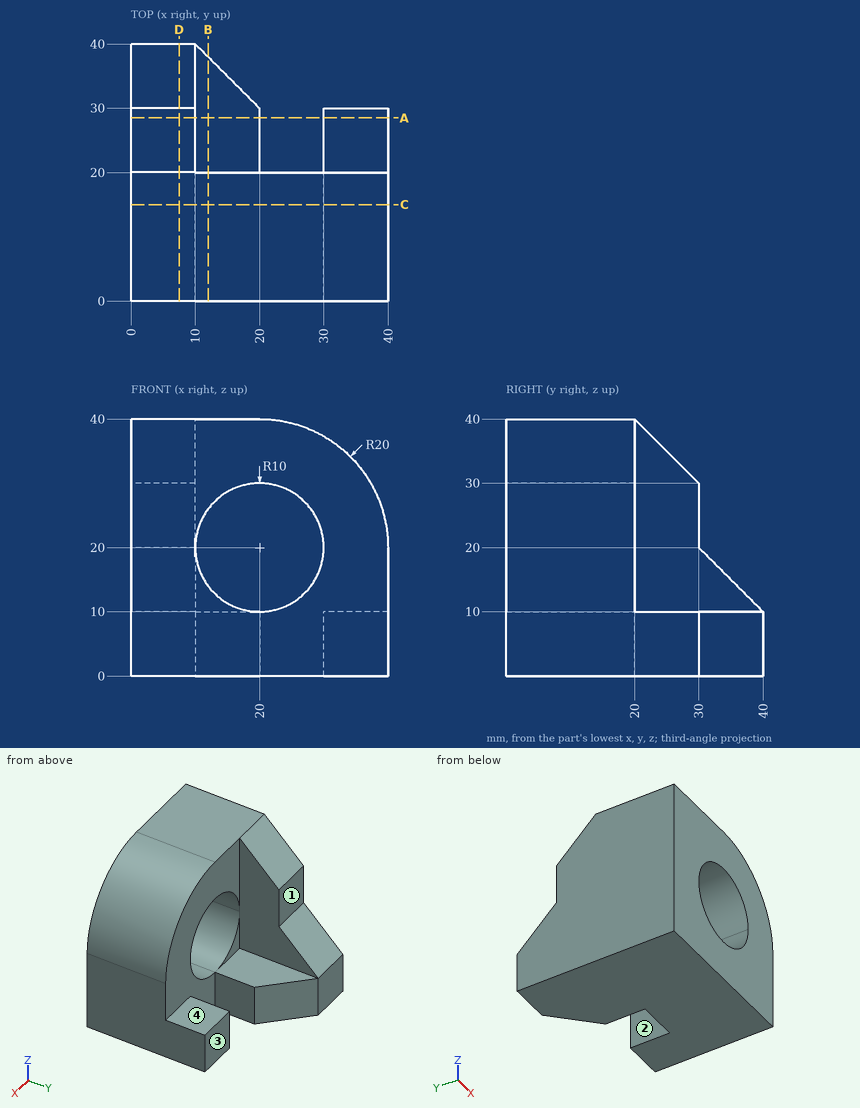
For this review, use the dimensioned drawing (mm, ordinates from the lowest corner) and the shaded views. A direction names the side the tool comes from. Coordinates: 2 decimals unless noted, no trailing zeros. Loops run counter-clockwise (first coordinate to the right, second up) from the corner with the lowest first, then second, coordinate; pieces in that order, holes last. Notation, with made-up numbers: (-13.5, 58.25) -> (6.5, 58.25) arc R33 cw to (6.5, 91.25) -> close; hole circle Ø7 at (-13.75, -17). An arc over 180 degrees is marked (long way). Use a Markdown table: item, result. Add a question column.
1. Add section B-B on x = 12. Write out the cut boundary in (y, z), plus the area to 3 significant figures.
2. Clearance check with flat-ended pins moving along their axes: pin 1 Ø11 at (x, z) = (7.5, 23.5) entering from +Y; pin 2 Ø6 at (x, y) = (7.5, 32) entering from +Z; pin 3 Ø8 at (x, z) = (15.5, 13) entering from +Y; pin 4 Ø6 at (y, z) = (35, 22) entering from +X. State where each tip first meets the part, or that it passes through.
3. Add section C-C on y = 15. Write out the cut boundary in (x, z), plus the area to 3 significant figures.
4. To check wall thickness, follow line 1 (X direction, y = 24, z = 8); line 2 (Z direction, x = 37, y = 20.5); line 3 (Y direction, x = 30.5, z = 36). State the ranges of each line that lie inside material, in increasing order.
5. Add section A-A on y = 28.5. Write out the cut boundary in (x, z), plus the area to 3 significant figures.
6. Add section D-D on x = 7.5. Write out the cut boundary in (y, z), plus the area to 3 significant figures.
7. Machinability: for the marked faces 1, 2, 3 and 4, which of the approach directions +Z, -Z, +X, -X, +Y, -Y give a long, thin tool a straight path to every point of the face, cutting with its end or side? Answer none if there is none.
Returned:
| question | item | result |
|---|---|---|
| 1 | outline | (0, 0) -> (38, 0) -> (38, 10) -> (20, 10) -> (20, 14) -> (0, 14) -> close; (0, 26) -> (20, 26) -> (20, 40) -> (0, 40) -> close |
| 1 | area | 740 mm² |
| 2 | pin 1 | stops at y = 32 |
| 2 | pin 2 | stops at z = 31 |
| 2 | pin 3 | stops at y = 37.15 |
| 2 | pin 4 | passes through |
| 3 | outline | (0, 0) -> (40, 0) -> (40, 20) arc R20 ccw to (20, 40) -> (0, 40) -> close; hole circle Ø20 at (20, 20) |
| 3 | area | 1,200 mm² |
| 4 | line 1 | x = 0 to 20, 30 to 40 |
| 4 | line 2 | z = 0 to 10 |
| 4 | line 3 | y = 0 to 20 |
| 5 | outline | (0, 0) -> (20, 0) -> (20, 10) -> (10, 10) -> (10, 31.5) -> (0, 31.5) -> close; (30, 0) -> (40, 0) -> (40, 10) -> (30, 10) -> close |
| 5 | area | 515 mm² |
| 6 | outline | (0, 0) -> (40, 0) -> (40, 10) -> (30, 20) -> (30, 30) -> (20, 40) -> (0, 40) -> close |
| 6 | area | 1,300 mm² |
| 7 | face 1 | +Z, +X, -X, +Y |
| 7 | face 2 | +Z, -Z, +Y |
| 7 | face 3 | +Z, -Z, +X, +Y |
| 7 | face 4 | +Z, +X, +Y |
